Design review of the part built by this model. Coordinates are the model's own, in mm. A direction names the side the tool comes from. Coordinates: 2 decimals unless noted, no trailing zeros. Write each loop counter-clockwise with the first axis right and the second up, starting at its lowest first coordinate (ties: lowest second). Pieces come first, ordered by that corner, then holes.
Q1. Take a section at B-B, the plane x = -10. Write out the cut boundary in (y, z), plus the area to 3 significant figures.
Q2. For L1, parallel to Y at x = 0, z = -5.25; L2, parallel to Z at x = 3.5, y = -7; L3, parallel to Y at x = 10.5, z = 3.5, list the stretches that pass through material, from the lowest coordinate up.
Q3. For faces 1 (the cylindrical face through (-7.08, -4.65, 1.57)), 2 (the cylindrical face through (-4.633, -6.184, 0.944)), list the 3-axis set-ups (+Z, -Z, +X, -X, +Y, -Y) from which the entire face can be reached by the end or side of a thin tool; tool diameter is ignored.
Q4. Take a section at D-D, the plane z = -10.5. Write out the cut boundary in (x, y).
Q5. Take a section at C-C, the plane x = 8.5. Write out the cut boundary in (y, z).
Q6. Take a section at A-A, the plane y = -7.25. Write out the cut boundary in (x, z), plus the area to 3 significant figures.
Q7. For pin 1 Ø3 at (x, z) = (-5, -8.66) entering from -Y; pin 2 Ø2 at (y, z) = (-4, -6.5) entering from +X; pin 3 Ø1.5 at (x, y) = (-4.5, -4.5) entering from +Z, all flat-tipped, find the tip position at first contact; note any pin that passes through.
Q8. The part is to be moulded in two halves that separate along X. For faces 3 (the cylindrical face through (-4.7, 0.018, -7.706)), 4 (the flat face through (-10.26, 0.31, -6.03)), 5 (the flat face through (10.09, -0.954, -5.715)), say which applies: released by +X, released by -X, zero draft, split by the parting line, or undercut.
from build123d import *

# Parameters (mm, degrees)
EXTRUDE_1_DEPTH          = 1.25
SKETCH_2_R               = 7.25
EXTRUDE_2_DEPTH          = 7.5
SKETCH_3_R               = 1.5
CUT_EXTRUDE_1_DEPTH      = 32.199772969
PATTERN_CIRCULAR_1_COUNT = 3
CHAMFER_1_SIZE           = 0.6
SKETCH_4_R               = 1
CUT_EXTRUDE_2_DEPTH      = 21.746646315


with BuildPart() as part:
    # 草图1 → 凸台-拉伸1 (new, symmetric)
    with BuildSketch(Plane(origin=(0, 0, 0), x_dir=(1, 0, 0), z_dir=(0, 1, 0))):
        Polygon((13.740936407, 0), (6.870468203, 11.9), (-6.870468203, 11.9), (-13.740936407, 0), (-6.870468203, -11.9), (6.870468203, -11.9), align=None)
    extrude(amount=EXTRUDE_1_DEPTH, both=True)

    # 草图2 → 凸台-拉伸2 (add)
    with BuildSketch(Plane.XZ.offset(1.25)):
        with Locations(Location((0, 0, 0), (0, 0, 270))):
            Circle(SKETCH_2_R)
    extrude(amount=EXTRUDE_2_DEPTH)

    # 草图3 → 切除-拉伸1 (cut, through all)
    with BuildSketch(Plane(origin=(-10.305702305, 0, 5.95), x_dir=(0.5000000000000071, 0, 0.8660254037844346), z_dir=(-0.8660254037844346, 0, 0.5000000000000071))):
        with Locations((0, -6.25)):
            Circle(SKETCH_3_R)
    cut_extrude_1 = extrude(amount=-CUT_EXTRUDE_1_DEPTH, mode=Mode.SUBTRACT)

    # 阵列(圆周)1: 切除-拉伸1 ×3 about axis
    pattern_circular_1_axis = Axis((0, -8.75, 0), (0, -1, 0))
    for i in range(1, PATTERN_CIRCULAR_1_COUNT):
        add(cut_extrude_1.rotate(pattern_circular_1_axis, i * 360 / PATTERN_CIRCULAR_1_COUNT), mode=Mode.SUBTRACT)

    # 倒角1
    chamfer_1_edges = [part.edges().sort_by_distance(p)[0] for p in [
        (0, -8.75, 7.25),
        (0, -1.25, 11.9),
        (-10.305702305, -1.25, 5.95),
        (-10.305702305, -1.25, -5.95),
        (0, -1.25, -11.9),
        (10.305702305, -1.25, -5.95),
        (10.305702305, -1.25, 5.95),
    ]]
    chamfer(chamfer_1_edges, length=CHAMFER_1_SIZE)

    # 草图4 → 切除-拉伸2 (cut, through all)
    with BuildSketch(Plane(origin=(0, 1.25, 0), x_dir=(1, 0, 0), z_dir=(0, 1, 0))):
        with Locations(Location((5, 8.660254038, 0), (0, 0, 270))):
            Circle(SKETCH_4_R)
        with Locations(Location((10, 0, 0), (0, 0, 270))):
            Circle(SKETCH_4_R)
        with Locations(Location((5, -8.660254038, 0), (0, 0, 270))):
            Circle(SKETCH_4_R)
        with Locations(Location((-5, -8.660254038, 0), (0, 0, 270))):
            Circle(SKETCH_4_R)
        with Locations(Location((-10, 0, 0), (0, 0, 270))):
            Circle(SKETCH_4_R)
        with Locations(Location((-5, 8.660254038, 0), (0, 0, 270))):
            Circle(SKETCH_4_R)
    extrude(amount=-CUT_EXTRUDE_2_DEPTH, mode=Mode.SUBTRACT)


solid = part.part
Responses:
1. outline: (-1.25, -5.28) - (-0.65, -6.48) - (1.25, -6.48) - (1.25, -1) - (-1.25, -1) - close; (-1.25, 1) - (1.25, 1) - (1.25, 6.48) - (-0.65, 6.48) - (-1.25, 5.28) - close
1. area: 26.7 mm2
2. L1: y = -8.75 to -7.75, -4.75 to 1.25
2. L2: z = -6.35 to -3.52, -0.52 to 0.52, 3.52 to 6.35
2. L3: y = -1.25 to 1.25
3. face 1: -Y
3. face 2: none
4. outline: (-7.68, -0.65) - (-6.99, -1.25) - (6.99, -1.25) - (7.68, -0.65) - (7.68, 1.25) - (-7.68, 1.25) - close
5. outline: (-1.25, -7.88) - (-0.65, -9.08) - (1.25, -9.08) - (1.25, 9.08) - (-0.65, 9.08) - (-1.25, 7.88) - close
6. outline: (-6.76, -2.61) - (-2.24, 0) - (-6.76, 2.61) arc R7.25 ccw to start; (-5.64, -4.55) arc R7.25 ccw to (-1.12, -7.16) - (-1.12, -1.94) - close; (-5.64, 4.55) - (-1.12, 1.94) - (-1.12, 7.16) arc R7.25 ccw to start; (1.12, -7.16) arc R7.25 ccw to (5.64, -4.55) - (1.12, -1.94) - close; (1.12, 1.94) - (5.64, 4.55) arc R7.25 ccw to (1.12, 7.16) - close; (2.24, 0) - (6.76, -2.61) arc R7.25 ccw to (6.76, 2.61) - close
6. area: 81.2 mm2
7. pin 1: stops at y = -1.25
7. pin 2: stops at x = 4.72
7. pin 3: stops at z = 6.2
8. face 3: undercut
8. face 4: released by -X
8. face 5: released by +X
